from build123d import *

# Parameters (mm, degrees)
CROQUIS1_W                  = 225
CROQUIS1_H                  = 220
SALIENTE_EXTRUIR1_DEPTH     = 120
CROQUIS2_W                  = 205
CROQUIS2_H                  = 210
CORTAR_EXTRUIR1_DEPTH       = 110
CROQUIS3_W                  = 30
CROQUIS3_H                  = 10
SALIENTE_EXTRUIR2_DEPTH     = 55
NERVIO4_REACH               = 276.693
CROQUIS6_WALL_W             = 587.44153369
CROQUIS6_WALL_H             = 30
SALIENTE_EXTRUIR3_DEPTH     = 65
SALIENTE_EXTRUIR4_START     = -15
SALIENTE_EXTRUIR4_OUTLINE_W = 40
SALIENTE_EXTRUIR4_OUTLINE_H = 27
SALIENTE_EXTRUIR4_DEPTH     = 52.5
CORTAR_EXTRUIR2_REACH       = 332.189
CROQUIS10_W                 = 30
CROQUIS10_H                 = 20
CORTAR_EXTRUIR3_REACH       = 276.693
CROQUIS11_W                 = 22
CROQUIS11_H                 = 17


with BuildPart() as part:
    # Croquis1 → Saliente-Extruir1 (new body)
    with BuildSketch(Plane.XY):
        with Locations((0, 110)):
            Rectangle(CROQUIS1_W, CROQUIS1_H)
    extrude(amount=SALIENTE_EXTRUIR1_DEPTH)

    # Croquis2 → Cortar-Extruir1 (cut)
    with BuildSketch(Plane.XY.offset(120)):
        with Locations((0, 115)):
            Rectangle(CROQUIS2_W, CROQUIS2_H)
    extrude(amount=-CORTAR_EXTRUIR1_DEPTH, mode=Mode.SUBTRACT)

    # Croquis3 → Saliente-Extruir2 (add)
    with BuildSketch(Plane.XY.offset(10)):
        with Locations((0, 65)):
            Rectangle(CROQUIS3_W, CROQUIS3_H)
    extrude(amount=SALIENTE_EXTRUIR2_DEPTH)

    # Croquis6 wall → Nervio4 (add, up to next)
    with BuildSketch(Plane(origin=(0, 50, 25), x_dir=(0, -0.554700196225, -0.832050294338), z_dir=(0, 0.832050294338, -0.554700196225)), mode=Mode.PRIVATE) as nervio4_sk1:
        Rectangle(CROQUIS6_WALL_W, CROQUIS6_WALL_H)
    nervio4_tool1 = extrude(nervio4_sk1.sketch, amount=NERVIO4_REACH, mode=Mode.PRIVATE) - part.part
    add(nervio4_tool1.solids().sort_by_distance((0, 50, 25))[0])



with BuildPart() as body_2:
    # Croquis7 → Saliente-Extruir3 (new body)
    with BuildSketch(Plane(origin=(0, 160, 0), x_dir=(1, 0, 0), z_dir=(0, 1, 0))):
        with BuildLine():
            Line((-40, -50), (-40, -10))
            Line((-40, -10), (0, -10))
            Line((0, -10), (40, -10))
            Line((40, -10), (40, -50))
            ThreePointArc((40, -50), (36.331804249, -66.733200531), (26, -80.397368307))
            Line((26, -80.397368307), (24.375, -78.497532788))
            ThreePointArc((24.375, -78.497532788), (0, -12.5), (-24.375, -78.497532788))
            Line((-24.375, -78.497532788), (-26, -80.397368307))
            ThreePointArc((-26, -80.397368307), (-36.331804249, -66.733200531), (-40, -50))
        make_face()
    extrude(amount=-SALIENTE_EXTRUIR3_DEPTH)


with BuildPart() as part_1:
    add(part.part)

    add(body_2.part)  # Saliente-Extruir4 merges body 2
    # Saliente-Extruir4: read off the stored shape, not the designer's step
    # Saliente-Extruir4 outline → Saliente-Extruir4 (add)
    with BuildSketch(Plane.YZ.offset(SALIENTE_EXTRUIR4_START)):
        with Locations((115, 23.5)):
            Rectangle(SALIENTE_EXTRUIR4_OUTLINE_W, SALIENTE_EXTRUIR4_OUTLINE_H)
    extrude(amount=SALIENTE_EXTRUIR4_DEPTH)

    # Croquis10 → Cortar-Extruir2 (cut, up to next)
    with BuildSketch(Plane.ZY.offset(-102.5), mode=Mode.PRIVATE) as cortar_extruir2_sk1:
        with Locations((88, 20)):
            Rectangle(CROQUIS10_W, CROQUIS10_H)
    cortar_extruir2_tool1 = extrude(cortar_extruir2_sk1.sketch, amount=-CORTAR_EXTRUIR2_REACH, mode=Mode.PRIVATE) & part_1.part
    add(cortar_extruir2_tool1.solids().sort_by_distance((102.5, 20, 88))[0], mode=Mode.SUBTRACT)

    # Croquis11 → Cortar-Extruir3 (cut, up to next)
    with BuildSketch(Plane(origin=(0, 0, 0), x_dir=(-1, 0, 0), z_dir=(0, 0, -1)), mode=Mode.PRIVATE) as cortar_extruir3_sk1:
        with Locations((-72.5, 30)):
            Rectangle(CROQUIS11_W, CROQUIS11_H)
    cortar_extruir3_tool1 = extrude(cortar_extruir3_sk1.sketch, amount=-CORTAR_EXTRUIR3_REACH, mode=Mode.PRIVATE) & part_1.part
    add(cortar_extruir3_tool1.solids().sort_by_distance((72.5, 30, 0))[0], mode=Mode.SUBTRACT)


solid = part_1.part
Source: CAD feature listing. Evaluate the final solid. Frame: model axes, mm. A direction names the side the tool comes from. Round coordinates to 2 decimals unless told otherwise and drop trailing zeros. Loops run counter-clockwise (first coordinate to the right, second up) from the corner with the lowest first, then second, coordinate; pieces in that order, holes last. Notation, with made-up numbers: M -20.5,79 L -11.5,79 A21 cw -11.5,86 Z; hole C 46.25,-3.5 d1. An arc over 180 degrees is marked long. Return JSON: item names as keys, results as strings. Group by question number.
1. Section query A-A on y = 122. Output: boundary loops of the cut face in (x, z) (3 decimals).
2. Section query C-C on y = 168. Output: boundary loops of the cut face in (x, z), and give its area (3 significant figures).
3. Section query B-B on x = 0. Output: boundary loops of the cut face in (y, z), and give its area (3 significant figures).
4. Material intervals for line 1 along X through (y, z) = (120.5, 50); line 2 along X through (y, z) = (51, 33); line 3 along Y through (x, z) = (-31, 20.5), sorted ascending. Write a range as from..to.
5. Pin query (flat end, axial travel): pin 1 (10 mm diameter, centred on x = -4, z = 16.5, fed in from -Y); pin 2 (4 mm diameter, centred on x = -69.5, z = 45.5, fed in from +Y); pin 3 (20 mm diameter, centred on x = 13, y = 108, fed in from +Z); pin 4 (5 mm diameter, centred on x = 54, y = 143, fed in from +Z). Return the tip coordinate at first contact, or that it passes through.
6. Mould query, pull axis X, two halves, no side actions, for faces 1 (the face through (102.5, 114, 66)), 2 (the face through (-2, 0, 59)). Classes: released by +X, released by -X, zero draft, split by the parting line, or undercut.
7. Reachability of faces 3 (the face through (0, 70, 37)), 4 (the face through (107, 20, 103)), 5 (the face through (-15, 115, 26)), 6 (the face through (83.5, 30, 5)), 7 (the face through (-9, 220, 6)) from +Z, -Z, +X, -X, +Y, -Y: full face, straight path, thin tool, end or side. Return the list, or none.
Checks:
{
 "1": {"outline": "M -112.5,0 L 112.5,0 L 112.5,120 L 102.5,120 L 102.5,10 L 40,10 L 40,50 A40 ccw 26,80.397 L 24.375,78.498 A37.5 cw 35.175,37 L -15,37 L -15,15.631 A37.5 cw -24.375,78.498 L -26,80.397 A40 ccw -40,50 L -40,10 L -102.5,10 L -102.5,120 L -112.5,120 Z"},
 "2": {"outline": "M -112.5,0 L 112.5,0 L 112.5,120 L 102.5,120 L 102.5,10 L -102.5,10 L -102.5,120 L -112.5,120 Z", "area": "4,450 mm²"},
 "3": {"outline": "M 0,0 L 220,0 L 220,10 L 160,10 L 160,12.5 L 135,12.5 L 135,37 L 95,37 L 95,10 L 70,10 L 70,65 L 60,65 L 60,40 L 40,10 L 10,10 L 10,120 L 0,120 Z", "area": "5,290 mm²"},
 "4": {"line 1": "x = -112.5..-102.5, -40..-37.5, 37.5..40, 102.5..112.5", "line 2": "x = -112.5..-102.5, 102.5..112.5", "line 3": "y = 0..10, 95..160"},
 "5": {"pin 1": "stops at y = 0", "pin 2": "stops at y = 10", "pin 3": "stops at z = 37", "pin 4": "stops at z = 10"},
 "6": {"face 1": "undercut", "face 2": "zero draft"},
 "7": {"face 3": "+Z", "face 4": "+X", "face 5": "+Z, +Y", "face 6": "+Z, -Z", "face 7": "+Z, -Z, +X, -X, +Y"}
}
